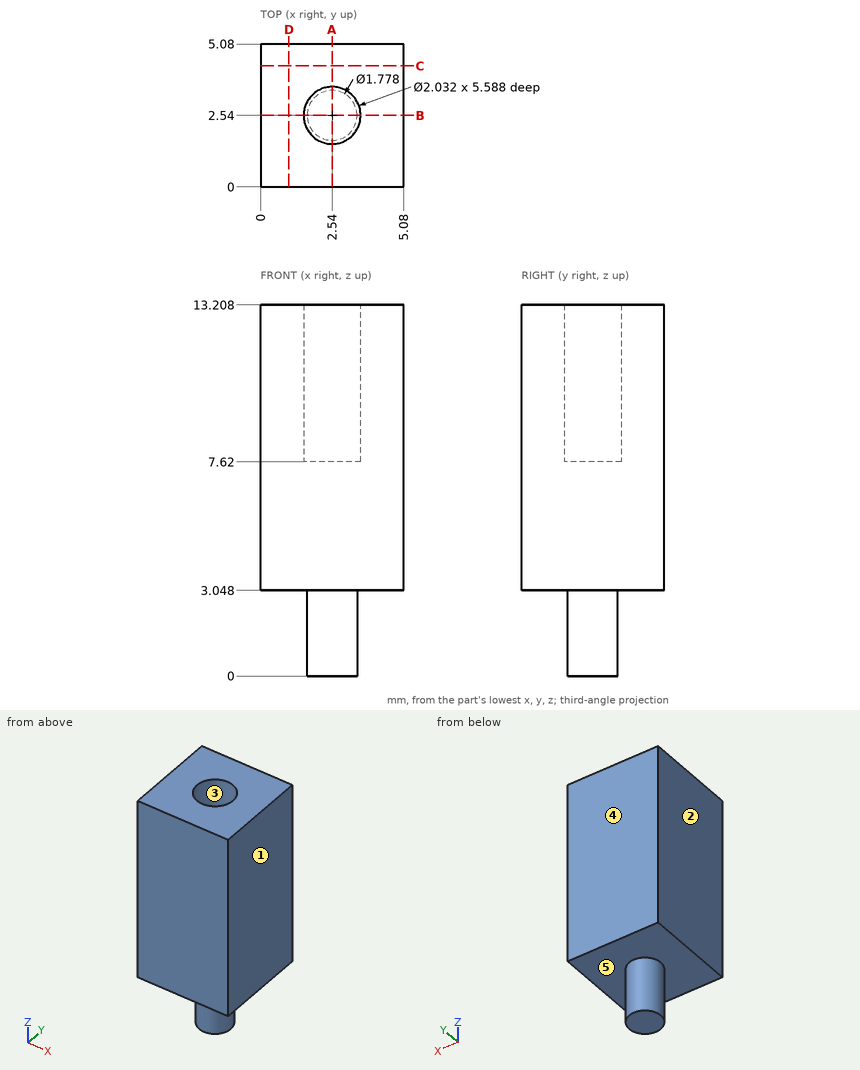
Could you check a few things on this drawing? It's one solid part, dimensions in mm from its lowest x, y, z. A direction names the side the tool comes from. Coordinates: 2 decimals unless noted, no trailing zeros. Loops run counter-clockwise (first coordinate to the right, second up) from the corner with the lowest first, then second, coordinate; pieces in that order, holes last. Notation, with made-up numbers: (-22.75, -30.75) - (-17.75, -30.75) arc R35 cw to (-17.75, 8.25) - close; hole circle Ø6 at (27.5, 49.25). An arc over 180 degrees is marked (long way). Answer as a JSON object with one key per item and string values. Group by question number.
Item 1: If we section it at A-A (x = 2.54): List the corners of the cut face in (y, z) for me.
Item 2: If I drill on L1, parallel to Y at x = 2.54, z = 9.95; L2, parallel to Z at x = 0.6, y = 2.5; L3, parallel to Y at x = 1.9, z = 7.75, over which ranges is the centre line in solid material (lowest first)? Write a range as from..to.
Item 3: If we section it at C-C (y = 4.3): List the corners of the cut face in (x, z) for me.
Item 4: For pin 1 (2 mm diameter, centred on x = 2.5, y = 3.5, fed in from -Z), with a flat end and sliding along its axis, tell me the tip position at first contact or that it passes through.
Item 5: If we mould it in two halves opening along X, with no side actions, what happens to the marked faces 1, 2 and 3? For each: released by +X, released by -X, zero draft, split by the parting line, or undercut.
Item 6: On a 3-axis mill with a long thin cutter (end or side, diameter ignored), from which of +Z, -Z, +X, -X, +Y, -Y can I reach the whole of each face in a straight line? I mean the marked faces 4 and 5. Say none if no direction works.
Returned:
{
 "1": {"outline": "(0, 3.05) - (1.65, 3.05) - (1.65, 0) - (3.43, 0) - (3.43, 3.05) - (5.08, 3.05) - (5.08, 13.21) - (3.56, 13.21) - (3.56, 7.62) - (1.52, 7.62) - (1.52, 13.21) - (0, 13.21) - close"},
 "2": {"L1": "y = 0..1.52, 3.56..5.08", "L2": "z = 3.05..13.21", "L3": "y = 0..1.75, 3.33..5.08"},
 "3": {"outline": "(0, 3.05) - (5.08, 3.05) - (5.08, 13.21) - (0, 13.21) - close"},
 "4": {"pin 1": "stops at z = 0"},
 "5": {"face 1": "released by +X", "face 2": "released by -X", "face 3": "undercut"},
 "6": {"face 4": "+Z, -Z, +X, -X, +Y", "face 5": "-Z"}
}
